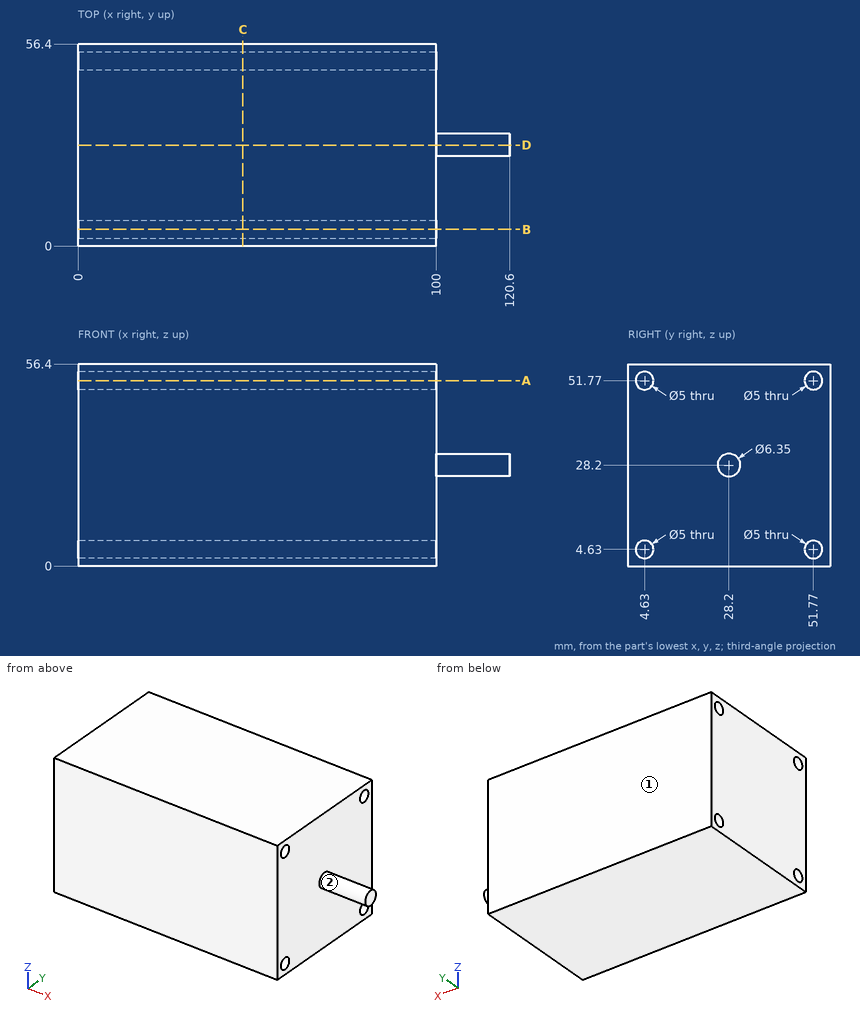
Can you work these out from the drawing? Everything is in mm from the part's minimum corner. A direction names the side the tool comes from. Give positions to 0.01 mm unless a question says otherwise; leave off trailing zeros. Order: outer loops, then holes, each group sorted by start corner. A loop starts at its lowest first (then second) coordinate and runs counter-clockwise, first axis right, second up.
1. For the marked faces 1 and 2, which set-ups out of +Z, -Z, +X, -X, +Y, -Y let a thin tool reach every point of the face, with its end or its side?
2. Will this pin go through, and if not, where does the flat tip stop? P1, Ø1.5, axis at y = 27, z = 19, coming from the +X side.
3. Suppose I cut it at C-C (x = 46). List the corners of the cut face in (y, z) for me.
4. Suppose I cut it at A-A (z = 51.77). List the corners of the cut face in (x, y) for me, plus the area to 3 significant figures.
5. Suppose I cut it at D-D (y = 28.2). List the corners of the cut face in (x, z) for me (3 decimals), plus the area to 3 significant figures.
6. I need wall thicknesses on L1, parallel to Y at x = 62.5, z = 51.77; L2, parallel to Y at x = 62, z = 4; L3, parallel to Z at x = 36, y = 51. Which ranges of each line are inside material? Lowest first, please.
Solved:
1. face 1: +Z, -Z, +X, -X, +Y
1. face 2: +X
2. P1: stops at x = 100
3. outline: (0, 0) - (56.4, 0) - (56.4, 56.4) - (0, 56.4) - close; hole circle Ø5 at (4.63, 4.63); hole circle Ø5 at (4.63, 51.77); hole circle Ø5 at (51.77, 4.63); hole circle Ø5 at (51.77, 51.77)
4. outline: (0, 0) - (100, 0) - (100, 2.13) - (0, 2.13) - close; (0, 7.13) - (100, 7.13) - (100, 49.27) - (0, 49.27) - close; (0, 54.27) - (100, 54.27) - (100, 56.4) - (0, 56.4) - close
4. area: 4,640 mm2
5. outline: (0, 0) - (100, 0) - (100, 25.025) - (120.6, 25.025) - (120.6, 31.375) - (100, 31.375) - (100, 56.4) - (0, 56.4) - close
5. area: 5,770 mm2
6. L1: y = 0 to 2.13, 7.13 to 49.27, 54.27 to 56.4
6. L2: y = 0 to 2.21, 7.05 to 49.35, 54.19 to 56.4
6. L3: z = 0 to 2.25, 7.01 to 49.39, 54.15 to 56.4
